CAD build for the part. Positions are in the model's coordinates, mm. Give positions to 0.01 mm unless a question says otherwise; leave off trailing zeros. Write each loop counter-clockwise with the first axis right and the second up, starting at its lowest first coordinate (ties: lowest second). Pieces come first, ordered by that corner, then holes. Notation, with made-up numbers: (-25, 72.25) -> (2, 72.25) arc R23 cw to (2, 93.25) -> close; hole circle Ø10 at (86.25, -27). An arc over 180 degrees is marked (long way). Answer in a Markdown table with one row per item. Add a question column.
Autodesk Inventor part; units mm, degrees
ref_plane "YZ Plane" through (0, 0, 0) normal (1, 0, 0) x (0, 1, 0)
ref_plane "XZ Plane" through (0, 0, 0) normal (0, 1, 0) x (-1, 0, 0)
ref_plane "XY Plane" through (0, 0, 0) normal (0, 0, 1) x (1, 0, 0)
ref_plane "Work Plane1" through (7.2162, 6.7561, 0) normal (0, 0, 1) x (-0.4175, -0.9087, 0)
sketch "Sketch1" plane through (7.2162, 6.7561, 0) normal (0, 0, 1) x (-0.4175, -0.9087, 0)
  circle A0 centre (9.5108, 16.1864) radius 1
  circle A1 centre (25.0108, -5.3136) radius 1
  circle A2 centre (4.5108, -11.8136) radius 1
  line L0 (22.0108, -1.8136) -> (8.5108, -1.8136)
  line L1 (8.5108, -1.8136) -> (8.5108, 13.6864)
  line L2 (8.5108, 13.6864) -> (22.0108, 13.6864)
  line L3 (22.0108, 13.6864) -> (22.0108, -1.8136)
  line L4 (11.1138, 15.6864) -> (23.6484, 15.6864)
  line L5 (23.6484, 15.6864) -> (23.6484, -3.7858)
  line L6 (23.6484, -3.7858) -> (27.5108, -3.7858)
  line L7 (27.5108, -3.7858) -> (27.5108, -8.9631)
  line L8 (27.5108, -8.9631) -> (27.5108, -14.3136)
  line L9 (27.5108, -14.3136) -> (1.8108, -14.3136)
  line L10 (1.8108, -14.3136) -> (1.8108, -10.169)
  line L11 (1.8108, -10.169) -> (6.5484, -10.169)
  line L12 (6.5484, -10.169) -> (6.5484, 18.6864)
  line L13 (6.5484, 18.6864) -> (11.1138, 18.6864)
  line L14 (11.1138, 18.6864) -> (11.1138, 15.6864)
  point P0 (9.1519, -3.7364)
  dimension "d0" = 2
  dimension "d1" = 2
  dimension "d2" = 2
  dimension "d3" = 28
  dimension "d5" = 15.5
  dimension "d6" = 5
  dimension "d8" = 20.5
  dimension "d9" = 2.5
  dimension "d10" = 1
  dimension "d12" = 3
  dimension "d13" = 33
  dimension "d14" = 25.7
  dimension "d15" = 17.1
  dimension "d23" = 30.5
  dimension "d24" = 9
  dimension "d25" = 2.5
extrude "Extrusion1" add sketch "Sketch1" along normal blind 1
fillet "Fillet1" radius 1 7 edges at (21.4621, -6.996, 0.5) (19.556, -11.1444, 0.5) (16.83, -9.8919, 0.5) (-6.0973, -13.1521, 0.5) (-7.7098, -16.6617, 0.5) (-2.7802, 9.3562, 0.5) (-4.7582, 5.0513, 0.5)
properties part number "00_KES400_Bluray_Lens"
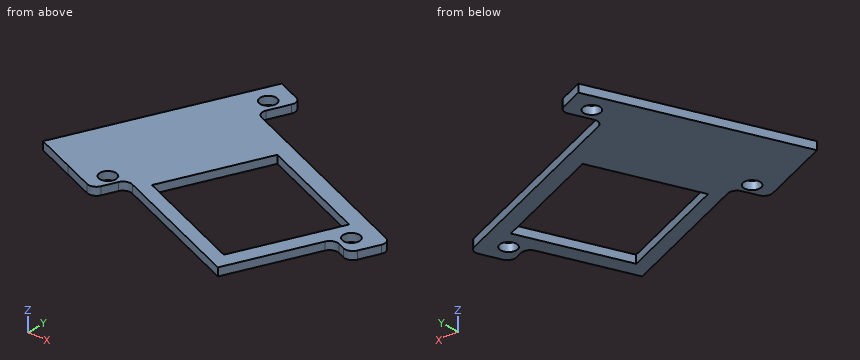
Item 1: Probe L1, parallel to X at y = -13, z = 0.5; L2, parallel to Y at x = 16, z = 0.25; L3, parallel to Y at x = 0, z = 0.1. List the from-to ranges inside material, lowest first. Write a range as from..to.
Item 2: Slice it at B-B, the plane x = -2. List the corners of the cut face in (y, z).
Item 3: Drop a flat-ended pin along its axis: pin 1 Ø2.5 at (x, y) = (17.95, -8.64) entering from -Z. Give the stop position or say it passes through.
Item 4: Slice it at D-D, the plane x = -11. List the corners of the cut face in (y, z), then the cut area to 3 significant figures.
Item 5: Slice it at A-A, the plane y = 7.5. List the corners of the cut face in (x, z), then the cut area to 3 significant figures.
Answer key:
| question | item | result |
|---|---|---|
| 1 | L1 | x = -15.68..-8.71, -7.4..-2.51, 13.2..15.4 |
| 1 | L2 | y = -11.7..-6.91, -6.65..-4.49 |
| 1 | L3 | y = -15.95..-14.15, -4.61..2.87 |
| 2 | outline | (-15.03, 0) -> (-13.23, 0) -> (-13.23, 1) -> (-15.03, 1) -> close; (-8.96, 0) -> (3.78, 0) -> (3.78, 1) -> (-8.96, 1) -> close |
| 3 | pin 1 | stops at z = 0 |
| 4 | outline | (-15.15, 0) -> (1.39, 0) -> (1.39, 1) -> (-15.15, 1) -> close |
| 4 | area | 16.5 mm² |
| 5 | outline | (-8.19, 0) -> (-6.4, 0) -> (-6.4, 1) -> (-8.19, 1) -> close; (-4.41, 0) -> (-3.63, 0) -> (-3.63, 1) -> (-4.41, 1) -> close |
| 5 | area | 2.57 mm² |
